Autodesk Inventor part; units mm, degrees
ref_plane "Work Plane1" through (-11.3, 27.1, 0) normal (1, 0, 0) x (0, 0, -1)
ref_plane "Work Plane3" through (-16.6, 27.1, -6.2) normal (-1, 0, 0) x (0, 0, 1)
ref_plane "YZ Plane" through (0, 0, 0) normal (1, 0, 0) x (0, 1, 0)
sketch "Sketch1" plane through (0, 0, 0) normal (0, 1, 0) x (-1, 0, 0)
  line L0 (0, 0) -> (22.6, 0)
  line L1 (22.6, 0) -> (22.6, -12.4)
  line L2 (22.6, -12.4) -> (0, -12.4)
  line L3 (0, -12.4) -> (0, 0)
  dimension "d0" = 22.6
  dimension "d1" = 12.4
extrude "Extrusion1" add sketch "Sketch1" along normal blind 27.1
sketch "Sketch2" plane through (0, 27.1, 0) normal (0, 1, 0) x (1, 0, 0)
  circle A0 centre (-16.6, 6.2) radius 2.4
  line L0 (-22.6, 12.4) -> (-22.6, 0)
  line L1 (-22.6, 0) -> (0, 0)
  line L2 (0, 12.4) -> (-22.6, 12.4)
  dimension "d4" = 4.8
  dimension "d5" = 6
  dimension "d6" = 6.2
  dimension "d7" = 6.2
extrude "Extrusion2" add sketch "Sketch2" along normal blind 3.1
sketch "Sketch3" plane through (0, 0, 0) normal (1, 0, 0) x (0, 0, -1)
  line L0 (0, 0) -> (0, 27.1)
  line L1 (12.4, 0) -> (12.4, 27.1)
  line L2 (0, 18.4) -> (12.4, 18.4)
  line L3 (12.4, 18.4) -> (12.4, 15.95)
  line L4 (12.4, 15.95) -> (0, 15.95)
  line L5 (0, 15.95) -> (0, 18.4)
  line L6 (0, 27.1) -> (12.4, 27.1)
  dimension "d10" = 2.45
  dimension "d11" = 8.7
extrude "Extrusion3" add sketch "Sketch3" along normal blind 4.85 contours L0 L2 L1 L4
ref_plane "Work Plane1" through (-11.3, 27.1, 0) normal (1, 0, 0) x (0, 0, -1)
mirror "Mirror1" about plane through (-11.3, 27.1, 0) normal (1, 0, 0) of "Extrusion3"
sketch "Sketch4" plane through (0, 18.4, 0) normal (0, 1, 0) x (1, 0, 0)
  circle A0 centre (2.6, 6.2) radius 1.05
  line L0 (-11.3, 14.88) -> (-11.3, -2.48)
  line L1 (0, 12.4) -> (4.85, 12.4)
  line L2 (0, 0) -> (4.85, 0)
  dimension "d14" = 2.1
  dimension "d15" = 13.9
  dimension "d16" = 6.2
  dimension "d17" = 6.2
extrude "Extrusion4" cut sketch "Sketch4" against normal through all
mirror "Mirror2" about plane through (-11.3, 27.1, 0) normal (1, 0, 0) of "Extrusion4"
ref_plane "Work Plane3" through (-16.6, 27.1, -6.2) normal (-1, 0, 0) x (0, 0, 1)
ref_plane "Work Plane2" through (-11.3, 27.1, 0) normal (1, 0, 0) x (0, 0, -1)
equation "\"d7\" = d6"
equation "\"d17\" = d16"
properties part number "servo"
The listing builds one solid part. Answer for the finished solid, in the listing's coordinates (mm). A direction names the side the tool comes from. Give positions to 0.01 mm unless a question says otherwise; leave off trailing zeros. Loops run counter-clockwise (first coordinate to the right, second up) from the corner with the lowest first, then second, coordinate; pieces in that order, holes last. Notation, with made-up numbers: (5, -27) - (43, -27) arc R28 cw to (43, 8) - close; hole circle Ø3 at (27.5, 32.5). An arc over 180 degrees is marked (long way). Write each question's results on one line, items separated by ' | '.
1. Which of the six approach directions +Z, -Z, +X, -X, +Y, -Y give full straight-line access (tool end or side, diameter ignored) to faces 1 (the face through (-24, 18.4, -6)), 2 (the face through (-24, 15.95, -6)), 3 (the face through (1, 18.4, -6))?
Resolved:
face 1: +Z, -Z, -X, +Y | face 2: +Z, -Z, -X, -Y | face 3: +Z, -Z, +X, +Y
2. Find section A-A, the plane x = -25.2. Write down the section's boundary in (y, z), then the cut area to 3 significant figures.
Resolved:
outline: (15.95, -12.4) - (18.4, -12.4) - (18.4, -7.25) - (15.95, -7.25) - close; (15.95, -5.15) - (18.4, -5.15) - (18.4, 0) - (15.95, 0) - close | area: 25.2 mm^2
3. Flat-ended cylindrical pins translate along their axes: P1, Ø1, axis at x = -6, z = -2.5, coming from the -Y side; P2, Ø5.5, axis at x = 1.5, z = -7, coming from the +Y side; P3, Ø3.5, axis at y = 9, z = -8, coming from the +X side; P4, Ø3.5, axis at x = 2.6, z = -6.2, coming from the +Y side. Find the tip coordinate at first contact, or state that the pin passes through.
Resolved:
P1: stops at y = 0 | P2: stops at y = 27.1 | P3: stops at x = 0 | P4: stops at y = 18.4
4. Consider probe 1 along X at (y, z) = (16.6, -6.2); probe 2 along Z at (x, y) = (-25.2, 16.8); probe 3 along Y at (x, z) = (-15.5, -2.75). Determine where each line is inside the solid, lowest interval first. Write a range as from..to.
Resolved:
probe 1: x = -27.45..-26.25, -24.15..1.55, 3.65..4.85 | probe 2: z = -12.4..-7.25, -5.15..0 | probe 3: y = 0..27.1
5. Find section C-C, the plane y = 18. Write down the section's boundary in (x, z), then the cut area to 3 significant figures.
Resolved:
outline: (-27.45, -12.4) - (4.85, -12.4) - (4.85, 0) - (-27.45, 0) - close; hole circle Ø2.1 at (-25.2, -6.2); hole circle Ø2.1 at (2.6, -6.2) | area: 394 mm^2
6. Find section D-D, the plane z = -11.25. Write down the section's boundary in (x, y).
Resolved:
outline: (-27.45, 15.95) - (-22.6, 15.95) - (-22.6, 0) - (0, 0) - (0, 15.95) - (4.85, 15.95) - (4.85, 18.4) - (0, 18.4) - (0, 27.1) - (-22.6, 27.1) - (-22.6, 18.4) - (-27.45, 18.4) - close
7. Find section B-B, the plane z = -6.2. Write down the section's boundary in (x, y), then the cut area to 3 significant figures.
Resolved:
outline: (-27.45, 15.95) - (-26.25, 15.95) - (-26.25, 18.4) - (-27.45, 18.4) - close; (-24.15, 15.95) - (-22.6, 15.95) - (-22.6, 0) - (0, 0) - (0, 15.95) - (1.55, 15.95) - (1.55, 18.4) - (0, 18.4) - (0, 27.1) - (-14.2, 27.1) - (-14.2, 30.2) - (-19, 30.2) - (-19, 27.1) - (-22.6, 27.1) - (-22.6, 18.4) - (-24.15, 18.4) - close; (3.65, 15.95) - (4.85, 15.95) - (4.85, 18.4) - (3.65, 18.4) - close | area: 641 mm^2
